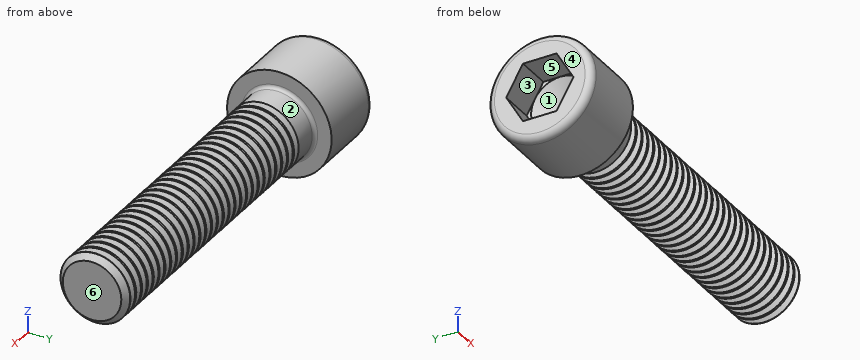
```python
from build123d import *

# Parameters (mm, degrees)
FILLET1_R       = 0.6
FILLET2_R       = 1.2
HEX_2_DEPTH     = 6
THDSCHPAT_COUNT = 29
THDSCHPAT_PITCH = 1.715517241


with BuildPart() as part:
    # BodySke → Base-Revolve (revolve)
    with BuildSketch(Plane.XY, mode=Mode.PRIVATE) as base_revolve_sk:
        Polygon((0, 0), (0, 9), (12, 9), (12, 6), (66.036, 6), (67, 5.036), (67, 0), align=None)
    revolve(base_revolve_sk.sketch.rotate(Axis((-31.75, 0, 0), (1, 0, 0)), 90), axis=Axis((-31.75, 0, 0), (1, 0, 0)))  # turned: the seam where the file's is

    # Fillet1
    fillet1_edges = [part.edges().sort_by_distance(p)[0] for p in [
        (12, 0, -6),
    ]]
    fillet(fillet1_edges, radius=FILLET1_R)

    # Fillet2
    fillet2_edges = [part.edges().sort_by_distance(p)[0] for p in [
        (0, 0, -9),
    ]]
    fillet(fillet2_edges, radius=FILLET2_R)

    # Sketch2 → Hex-PreBroach (revolve, cut)
    with BuildSketch(Plane.XY, mode=Mode.PRIVATE) as hex_prebroach_sk:
        Polygon((0, 5.0125), (6, 5.0125), (8.893968224, 0), (0, 0), align=None)
    revolve(hex_prebroach_sk.sketch.rotate(Axis((0, 0, 0), (1, 0, 0)), 90), axis=Axis((0, 0, 0), (1, 0, 0)), mode=Mode.SUBTRACT)  # turned: the seam where the file's is

    # Sketch3 → Hex 2 (cut)
    with BuildSketch(Plane(origin=(0, 0, 0), x_dir=(0, 0.5, 0.866025404), z_dir=(-1, 0, 0))):
        Polygon((2.893968224, 5.0125), (-2.893968224, 5.0125), (-5.787936449, 0), (-2.893968224, -5.0125), (2.893968224, -5.0125), (5.787936449, 0), align=None)
    extrude(amount=-HEX_2_DEPTH, mode=Mode.SUBTRACT)

    # ThdSchSke → ThreadSchematic (revolve, cut)
    with BuildSketch(Plane.XY, mode=Mode.PRIVATE) as threadschematic_sk:
        Polygon((17.25, -5.036), (16.574999933, -6), (16.574999933, -7.5), (17.925000067, -7.5), (17.925000067, -6), align=None)
    threadschematic = revolve(threadschematic_sk.sketch.rotate(Axis((-3.175, 0, 0), (1, 0, 0)), 270), axis=Axis((-3.175, 0, 0), (1, 0, 0)), mode=Mode.SUBTRACT)  # turned: the seam where the file's is

    # ThdSchPat: ThreadSchematic ×29
    with Locations(*[(i * THDSCHPAT_PITCH, 0, 0) for i in range(1, THDSCHPAT_COUNT)]):
        add(threadschematic, mode=Mode.SUBTRACT)


solid = part.part
```
The model under review builds one solid part; all positions refer to its coordinate system, in mm. Face numbers are marked on the shaded views. A direction names the side the tool comes from. Give positions to 0.01 mm unless a question says otherwise; leave off trailing zeros. Answer in a Markdown table with one row per item. Add a question column.
1. Draft analysis for pull direction Z (two halves, no side actions). For the marked faces 1, 2, 3 and 4, state which applies: +Z half, -Z half, draft (parallel to the pull), parting line (faces both ways), or undercut.
2. Tool access review of the marked faces 5 and 6: name each direction out of +Z, -Z, +X, -X, +Y, -Y from which nothing blocks a thin tool from reaching the whole face with its end or side.
3. Insertion check: P1, Ø4, axis at x = 11.5, y = -3.5, coming from the +Z side; P2, Ø1, axis at x = 43.5, y = 2.5, coming from the -Z side; P3, Ø2, axis at x = 36, z = -6, coming from the +Y side. Each pin has a flat end and moves straight along its axis. Give the tip position at first contact, or say it passes through.
4. Wall thickness on line 1 along X through (y, z) = (4, 6); line 2 along X through (y, z) = (-6, -1.5); line 3 along Y through (x, z) = (31.5, 1.25): over which ranges is each line inside the solid? List them lowest first. Write a range as [from, to].
Ans:
| question | item | result |
|---|---|---|
| 1 | face 1 | undercut |
| 1 | face 2 | parting line |
| 1 | face 3 | undercut |
| 1 | face 4 | draft |
| 2 | face 5 | -X |
| 2 | face 6 | +Z, -Z, +X, +Y, -Y |
| 3 | P1 | stops at z = 8.87 |
| 3 | P2 | stops at z = -5.65 |
| 3 | P3 | stops at y = 3.05 |
| 4 | line 1 | x = [0, 12] |
| 4 | line 2 | x = [0, 12.17] |
| 4 | line 3 | y = [-5.65, 5.65] |
